Input: part model. Units: mm. Frame: model coordinates. Round coordinates to 2 decimals unless told otherwise and drop trailing zeros. Loops run counter-clockwise (first coordinate to the right, second up) from the corner with the lowest first, then second, coordinate; pieces in that order, holes last.
1) First-contact query: pin 1 (4 mm diameter, centred on x = 16.68, y = 0, fed in from +Z); pin 2 (2 mm diameter, centred on x = 25.5, z = 2.5, fed in from -Y). Flat tips, straight axial feed; report the tip coordinate or a pass-through.
2) Ray query, line 1 along Y through (x, z) = (0, 2.4); line 2 along X through (y, z) = (1, 3.25); line 3 along Y through (x, z) = (40.5, 3.25). Return the intervals inside material, ascending.
3) Section C-C, the plane z = 2.7. Return loops of the section in (x, y).
4) Draft query along Y for faces 1 (the face through (-24.262, 0.11, 2.028)), 2 (the face through (-30, -20, 2)), 3 (the face through (-1, -6, 4)). Return one class per face: pulls with the +Y half, pulls with the -Y half, needs draft (parallel to the pull), parting line crosses it, or undercut.
5) Section B-B, the plane y = 0. Return loops of the section in (x, z), and give its area (3 significant figures).
6) Section A-A, the plane x = 0. Return loops of the section in (y, z), and give its area (3 significant figures).
from build123d import *

# Parameters (mm, degrees)
BOSS_EXTRUDE2_DEPTH = 4
SKETCH4_OUTSIDE_W   = 125.338
SKETCH4_OUTSIDE_H   = 85.338
SKETCH4_OUTSIDE_R   = 2.5
CUT_EXTRUDE4_DEPTH  = 4
FILLET1_R           = 0.15


with BuildPart() as part:
    # Sketch1 → Boss-Extrude2 (new body)
    with BuildSketch(Plane.XY):
        Polygon((-50, 10), (-50, -10), (-10, -30), (10, -30), (50, -10), (50, 10), (10, 30), (-10, 30), align=None)
    extrude(amount=BOSS_EXTRUDE2_DEPTH)

    # Sketch4 outside → Cut-Extrude4 (cut)
    with BuildSketch(Plane.XY.offset(4)):
        Rectangle(SKETCH4_OUTSIDE_W, SKETCH4_OUTSIDE_H)
        Polygon((-10, 30), (-50, 10), (-50, -10), (-10, -30), (10, -30), (50, -10), (50, 10), (10, 30), align=None, mode=Mode.SUBTRACT)
        Circle(SKETCH4_OUTSIDE_R)
        with Locations((-21.764530358, 0)):
            Circle(SKETCH4_OUTSIDE_R)
        with Locations((-42.602849817, 0)):
            Circle(SKETCH4_OUTSIDE_R)
        with Locations((16.676409958, 0)):
            Circle(SKETCH4_OUTSIDE_R)
        with Locations((39.134669841, 0)):
            Circle(SKETCH4_OUTSIDE_R)
        with Locations((0, 18.729540895)):
            Circle(SKETCH4_OUTSIDE_R)
        with Locations((0, -17.102871632)):
            Circle(SKETCH4_OUTSIDE_R)
    extrude(amount=-CUT_EXTRUDE4_DEPTH, mode=Mode.SUBTRACT)

    # Fillet1
    fillet1_edges = [part.edges().sort_by_distance(p)[0] for p in [
        (-30, -20, 4),
        (-50, 0, 0),
        (-30, 20, 0),
        (0, -30, 4),
        (-10, 30, 2),
        (10, 30, 2),
        (50, 10, 2),
        (50, -10, 2),
        (10, -30, 2),
        (-10, -30, 2),
        (-50, -10, 2),
        (-50, 10, 2),
        (30, -20, 4),
        (50, 0, 4),
        (30, 20, 4),
        (0, 30, 4),
        (-30, 20, 4),
        (-50, 0, 4),
        (0, 30, 0),
        (30, 20, 0),
        (50, 0, 0),
        (30, -20, 0),
        (0, -30, 0),
        (-30, -20, 0),
    ]]
    fillet(fillet1_edges, radius=FILLET1_R)


solid = part.part
Final values:
1. pin 1: passes through
1. pin 2: stops at y = -22.75
2. line 1: y = -30 to -19.6, -14.6 to -2.5, 2.5 to 16.23, 21.23 to 30
2. line 2: x = -50 to -44.89, -40.31 to -24.06, -19.47 to -2.29, 2.29 to 14.39, 18.97 to 36.84, 41.43 to 50
2. line 3: y = -14.75 to -2.09, 2.09 to 14.75
3. outline: (-50, -9.91) arc R0.15 ccw to (-49.92, -10.04) - (-10.03, -29.98) arc R0.15 ccw to (-9.96, -30) - (9.96, -30) arc R0.15 ccw to (10.03, -29.98) - (49.92, -10.04) arc R0.15 ccw to (50, -9.91) - (50, 9.91) arc R0.15 ccw to (49.92, 10.04) - (10.03, 29.98) arc R0.15 ccw to (9.96, 30) - (-9.96, 30) arc R0.15 ccw to (-10.03, 29.98) - (-49.92, 10.04) arc R0.15 ccw to (-50, 9.91) - close; hole circle Ø5 at (-42.6, 0); hole circle Ø5 at (-21.76, 0); hole circle Ø5 at (0, -17.1); hole circle Ø5 at (0, 0); hole circle Ø5 at (0, 18.73); hole circle Ø5 at (16.68, 0); hole circle Ø5 at (39.13, 0)
4. face 1: undercut
4. face 2: pulls with the -Y half
4. face 3: needs draft
5. outline: (-50, 0.15) arc R0.15 ccw to (-49.85, 0) - (-45.1, 0) - (-45.1, 4) - (-49.85, 4) arc R0.15 ccw to (-50, 3.85) - close; (-40.1, 0) - (-24.26, 0) - (-24.26, 4) - (-40.1, 4) - close; (-19.26, 0) - (-2.5, 0) - (-2.5, 4) - (-19.26, 4) - close; (2.5, 0) - (14.18, 0) - (14.18, 4) - (2.5, 4) - close; (19.18, 0) - (36.63, 0) - (36.63, 4) - (19.18, 4) - close; (41.63, 0) - (49.85, 0) arc R0.15 ccw to (50, 0.15) - (50, 3.85) arc R0.15 ccw to (49.85, 4) - (41.63, 4) - close
5. area: 300 mm2
6. outline: (-30, 0.15) arc R0.15 ccw to (-29.85, 0) - (-19.6, 0) - (-19.6, 4) - (-29.85, 4) arc R0.15 ccw to (-30, 3.85) - close; (-14.6, 0) - (-2.5, 0) - (-2.5, 4) - (-14.6, 4) - close; (2.5, 0) - (16.23, 0) - (16.23, 4) - (2.5, 4) - close; (21.23, 0) - (29.85, 0) arc R0.15 ccw to (30, 0.15) - (30, 3.85) arc R0.15 ccw to (29.85, 4) - (21.23, 4) - close
6. area: 180 mm2
